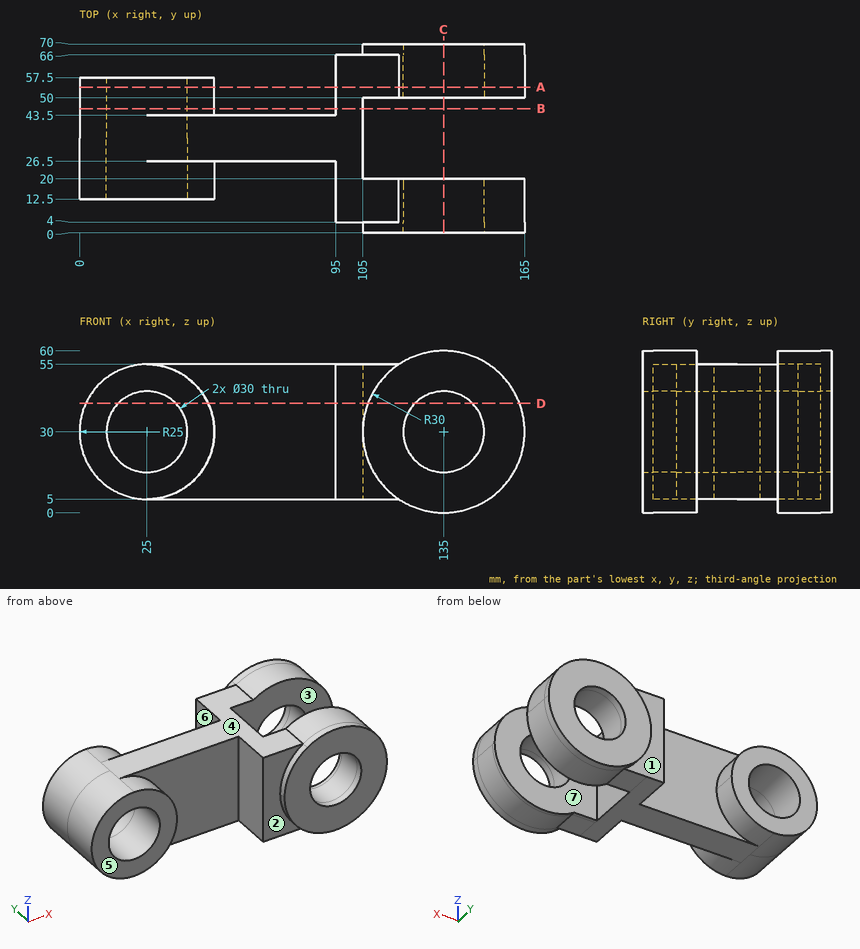
Study the drawing (mm; zero at the part's minimum x, y, z) and answer. A direction names the side the tool comes from. Give positions to 0.01 mm unless a question says otherwise; leave off trailing zeros. Order: outer loops, then holes, each group sorted by start corner. A loop starts at its lowest first (then second) coordinate and runs counter-clockwise, first axis right, second up.
1) Find section A-A on y = 54. Write down the section's boundary in (x, z), then the cut area to 3 significant figures.
Reported:
outline: circle Ø50 at (25, 30); (95, 5) - (118.42, 5) arc R30 ccw (long way) to (118.42, 55) - (95, 55) - close; hole circle Ø30 at (25, 30); hole circle Ø30 at (135, 30)
area: 4,080 mm2
2) Find section D-D on z = 40.5. Give the number of separate pieces and of enclosed holes in the cut face, then the cut area to 3 significant figures.
Reported:
separate pieces: 4
enclosed holes: 0
area: 3,950 mm2
3) Given P1, Ø5, axis at x = 47.5, z = 23.5, coming from the -Y side; P2, Ø18, axis at x = 25, z = 30, coming from the +Y side; P3, Ø25, axis at x = 71.5, z = 29.5, coming from the -Y side; P4, Ø18.5, axis at x = 75.5, y = 27.5, coming from the +Z side, each flat-ended and moving along its own axis, determine where each tip first touches the part or whether it passes through.
Reported:
P1: stops at y = 12.5
P2: passes through
P3: stops at y = 26.5
P4: stops at z = 55
4) Find section C-C on x = 135. Write down the section's boundary in (y, z), then the cut area to 3 significant figures.
Reported:
outline: (0, 0) - (20, 0) - (20, 15) - (0, 15) - close; (0, 45) - (20, 45) - (20, 60) - (0, 60) - close; (50, 0) - (70, 0) - (70, 15) - (50, 15) - close; (50, 45) - (70, 45) - (70, 60) - (50, 60) - close
area: 1,200 mm2
5) Determine the mould class of the marked faces 5, 6 and 7 for opening direction Y: pulls with the +Y half, pulls with the -Y half, needs draft (parallel to the pull), parting line crosses it, or undercut.
Reported:
face 5: pulls with the -Y half
face 6: needs draft
face 7: undercut
6) For the marked faces 1, 2, 3 and 4, determine the directions among +Z, -Z, +X, -X, +Y, -Y from which every point of the face is accessible in a straight line to the end or side of a thin tool.
Reported:
face 1: -X, +Y
face 2: -X, -Y
face 3: +Z, -Z, +X
face 4: +Z, -X, +Y, -Y
7) Find section B-B on y = 46. Write down the section's boundary in (x, z).
Reported:
outline: circle Ø50 at (25, 30); (95, 5) - (105, 5) - (105, 55) - (95, 55) - close; hole circle Ø30 at (25, 30)
8) Consider line 1 along X through (y, z) = (49.5, 30); line 2 along Z through (x, y) = (135, 68); line 3 along X through (y, z) = (50.5, 30). Determine where each line is inside the solid, lowest interval first.
Reported:
line 1: x = 0 to 10, 40 to 50, 95 to 105
line 2: z = 0 to 15, 45 to 60
line 3: x = 0 to 10, 40 to 50, 95 to 120, 150 to 165
